from build123d import *
from OCP.BRepAlgoAPI import BRepAlgoAPI_Cut
from OCP.TopTools import TopTools_ListOfShape

# Parameters (mm, degrees)
CUT_EXTRUDE_1_DEPTH      = 9.395352378
CUT_EXTRUDE_1_DEPTH_BACK = 9.395352378
SKETCH_2_W               = 3
SKETCH_2_H               = 3.541131468
EXTRUDE_START            = -2.0183
EXTRUDE_1_DEPTH          = 6
EXTRUDE_2_DEPTH          = 3
EXTRUDE_2_DEPTH_BACK     = 3
SKETCH_6_R               = 1.6
CUT_EXTRUDE_2_DEPTH      = 23.66980552
SKETCH_7_R               = 4
CUT_EXTRUDE_3_DEPTH      = 23.219551454
FILLET_1_R               = 2


with BuildPart() as part:
    # 草图1 → 旋转1 (revolve)
    with BuildSketch(Plane.XY, mode=Mode.PRIVATE) as revolve_1_sk:
        with BuildLine():
            Line((4, 3.981699636), (4, -2.018300364))
            Line((4, -2.018300364), (5, -2.018300364))
            ThreePointArc((5, -2.018300364), (5.226280067, 0.981699636), (5, 3.981699636))
            Line((5, 3.981699636), (4, 3.981699636))
        make_face()
    revolve(revolve_1_sk.sketch.rotate(Axis((0, -4.923271421, 0), (0, 1, 0)), 90), axis=Axis((0, -4.923271421, 0), (0, 1, 0)))

    # 草图2 → 切除-拉伸1 (cut, two sides: drawn at the far end of the back side and taken through both)
    with BuildSketch(Plane(origin=(0, 0, 0), x_dir=(1, 0, 0), z_dir=(0, 1, 0)).offset(-CUT_EXTRUDE_1_DEPTH_BACK)):
        with Locations((0, 5.060025588)):
            Rectangle(SKETCH_2_W, SKETCH_2_H)
    extrude(amount=CUT_EXTRUDE_1_DEPTH + CUT_EXTRUDE_1_DEPTH_BACK, mode=Mode.SUBTRACT)

    # 草图3 → 凸台-拉伸1 (add)
    with BuildSketch(Plane(origin=(0, 0, 0), x_dir=(1, 0, 0), z_dir=(0, 1, 0)).offset(EXTRUDE_START)):
        Polygon((-1.5, 3.708099244), (-0.5, 3.708099244), (-0.5, 11.708099244), (-1.5, 11.708099244), (-1.5, 4.981969012), align=None)
        Polygon((1.5, 11.708099244), (1.5, 4.981969012), (1.5, 3.708099244), (0.5, 3.708099244), (0.5, 11.708099244), align=None)
    extrude(amount=EXTRUDE_1_DEPTH)

    # 草图5 → 凸台-拉伸2 (add, two sides: drawn at the far end of the back side and taken through both)
    with BuildSketch(Plane(origin=(0, 0, 0), x_dir=(0, 0, -1), z_dir=(1, 0, 0)).offset(-EXTRUDE_2_DEPTH_BACK)):
        with BuildLine():
            Line((-3.745950378, 3.981699636), (-17.745950378, 3.981699636))
            ThreePointArc((-17.745950378, 3.981699636), (-20.745950378, 0.981699636), (-17.745950378, -2.018300364))
            Line((-17.745950378, -2.018300364), (-3.745950378, -2.018300364))
            Line((-3.745950378, -2.018300364), (-3.745950378, 3.981699636))
        make_face()
    extrude(amount=EXTRUDE_2_DEPTH + EXTRUDE_2_DEPTH_BACK)

    # 草图6 → 切除-拉伸2 (cut, through all)
    with BuildSketch(Plane(origin=(3, 0, 0), x_dir=(0, 0, -1), z_dir=(1, 0, 0))):
        with Locations((-17.745950378, 0.981699636)):
            Circle(SKETCH_6_R)
        with Locations((8.208099244, 0.981699636)):
            Circle(SKETCH_6_R)
        with Locations((-11.745950378, 0.981699636)):
            Circle(SKETCH_6_R)
    extrude(amount=-CUT_EXTRUDE_2_DEPTH, mode=Mode.SUBTRACT)


with BuildPart() as cut_extrude_3_tool:
    # 草图7 → 切除-拉伸3 (new, through all)
    with BuildSketch(Plane(origin=(0, 3.981699636, 0), x_dir=(1, 0, 0), z_dir=(0, 1, 0))):
        Circle(SKETCH_7_R)
    extrude(amount=-CUT_EXTRUDE_3_DEPTH)


with BuildPart() as part_1:
    add(part.part)

    # 切除-拉伸3: cut by cut_extrude_3_tool, with a tolerance
    cut_extrude_3_stock = TopTools_ListOfShape()
    cut_extrude_3_stock.Append(part_1.part.wrapped)
    cut_extrude_3_tools = TopTools_ListOfShape()
    cut_extrude_3_tools.Append(cut_extrude_3_tool.part.wrapped)
    cut_extrude_3_cut = BRepAlgoAPI_Cut()
    cut_extrude_3_cut.SetArguments(cut_extrude_3_stock)
    cut_extrude_3_cut.SetTools(cut_extrude_3_tools)
    cut_extrude_3_cut.SetFuzzyValue(0.00001)
    cut_extrude_3_cut.Build()
    add(Compound.cast(cut_extrude_3_cut.Shape()).solids(), mode=Mode.REPLACE)

    # 圆角1
    fillet_1_edges = [part_1.edges().sort_by_distance(p)[0] for p in [
        (-1, -2.0183, -11.708099244),
        (-1, 3.9817, -11.708099244),
        (1, -2.0183, -11.708099244),
        (1, 3.9817, -11.708099244),
    ]]
    fillet(fillet_1_edges, radius=FILLET_1_R)


solid = part_1.part
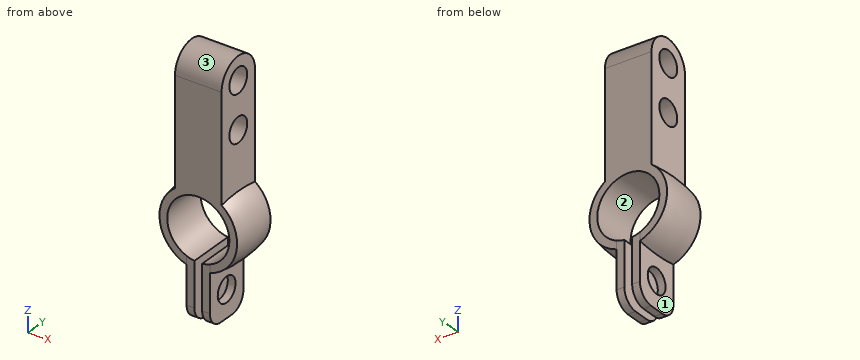
Verification items for the finished model (mm, model axes). Face numbers are marked on the shaded views. Coordinates: 2 decimals unless noted, no trailing zeros. Order: outer loops, then holes, each group sorted by start corner. A loop starts at its lowest first (then second) coordinate and runs counter-clockwise, first axis right, second up. Notation, with made-up numbers: (2, 62.5) -> (27, 62.5) arc R9 ccw to (27, 66.5) -> close; hole circle Ø6 at (87.5, 88.5). An arc over 180 degrees is marked (long way). Use CSV: the item, a comma, the result in double quotes. Start each with the question number.
Q1. Section check C-C, the plane x = 2.25. Give the number of separate pieces and of enclosed holes in the cut face, and give its area (3 significant figures).
Q2. Depth check by flat-ended pin: P1, Ø1.8, axis at y = 0.5, z = 12.5, coming from the -X side; P2, Ø3, axis at y = 0, z = -8.5, coming from the +X side. Enter the tip coordinate at first touch or a pass-through.
Q3. Section check D-D, the plane z = 15. Record the cut outline in (x, y), and give its area (3 significant figures).
Q4. Section check B-B, the plane x = 0. Record the cut outline in (y, z), and give its area (3 significant figures).
Q5. Thickness scan on line 1 along Z through (x, y) = (-1.75, 0); line 2 along Z through (x, y) = (-2.75, 2); line 3 along X through (y, z) = (0.75, 14). Record the ranges inside material, lowest first.
Q6. Section check A-A, the plane z = -5.5. Record the cut outline in (x, y), and give its area (3 significant figures).
Q7. Draft check along X on the marked faces 1, 2 and 3. Enter one of: +X half, -X half, draft (parallel to the pull), parting line (faces both ways), or undercut.
Returned:
1,separate pieces,"2"
1,enclosed holes,"2"
1,area,"92.6 mm^2"
2,P1,"stops at x = -3"
2,P2,"stops at x = 1.5"
3,outline,"(-3, -2.02) -> (3, -2.02) -> (3, 3.98) -> (-3, 3.98) -> close"
3,area,"36.0 mm^2"
4,outline,"(-2.02, 4) -> (3.98, 4) -> (3.98, 17.75) arc R3 ccw to (-2.02, 17.75) -> close; hole circle Ø3.2 at (0.98, 11.75); hole circle Ø3.2 at (0.98, 17.75)"
4,area,"80.5 mm^2"
5,line 1,"z = -4.9 to -3.6, 3.6 to 10.48, 13.01 to 16.48, 19.01 to 20.58"
5,line 2,"z = -4.41 to -2.9, 2.9 to 10.51, 12.98 to 16.51, 18.98 to 20.57"
5,line 3,"x = -3 to 3"
6,outline,"(-1.5, -2.02) -> (-0.5, -2.02) -> (-0.5, 3.98) -> (-1.5, 3.98) -> close; (0.5, -2.02) -> (1.5, -2.02) -> (1.5, 3.98) -> (0.5, 3.98) -> close"
6,area,"12.0 mm^2"
7,face 1,"-X half"
7,face 2,"undercut"
7,face 3,"draft"
